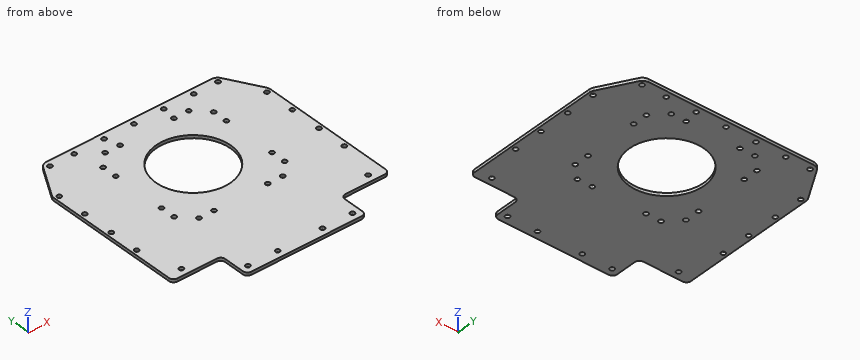
```python
from build123d import *

# Parameters (mm, degrees)
SKETCH_1_R          = 1.5
EXTRUDE_1_DEPTH     = 2
SKETCH_2_R          = 25
CUT_EXTRUDE_1_DEPTH = 2


with BuildPart() as part:
    # 草图1 → 凸台-拉伸1 (new body)
    with BuildSketch(Plane.XY):
        with BuildLine():
            Line((-60.191772409, 67.5), (-72.512280484, 46.160254038))
            ThreePointArc((-72.512280484, 46.160254038), (-73.011782597, 44.954349263), (-73.182153465, 43.660254038))
            Line((-73.182153465, 43.660254038), (-73.182153465, -47))
            ThreePointArc((-73.182153465, -47), (-72.303473809, -49.121320344), (-70.182153465, -50))
            Line((-70.182153465, -50), (-43.682153465, -50))
            ThreePointArc((-43.682153465, -50), (-41.560833122, -50.878679656), (-40.682153465, -53))
            Line((-40.682153465, -53), (-40.682153465, -67))
            ThreePointArc((-40.682153465, -67), (-39.803473809, -69.121320344), (-37.682153465, -70))
            Line((-37.682153465, -70), (36.317846535, -70))
            ThreePointArc((36.317846535, -70), (38.439166878, -69.121320344), (39.317846535, -67))
            Line((39.317846535, -67), (39.317846535, -53))
            ThreePointArc((39.317846535, -53), (40.196526191, -50.878679656), (42.317846535, -50))
            Line((42.317846535, -50), (68.817846535, -50))
            ThreePointArc((68.817846535, -50), (70.939166878, -49.121320344), (71.817846535, -47))
            Line((71.817846535, -47), (71.817846535, 43.660254038))
            ThreePointArc((71.817846535, 43.660254038), (71.647475666, 44.954349263), (71.147973554, 46.160254038))
            Line((71.147973554, 46.160254038), (58.827465478, 67.5))
            ThreePointArc((58.827465478, 67.5), (56.997338459, 69.330127019), (54.497338459, 70))
            Line((54.497338459, 70), (-55.86164539, 70))
            ThreePointArc((-55.86164539, 70), (-58.36164539, 69.330127019), (-60.191772409, 67.5))
        make_face()
        with Locations((-0.682153465, 66)):
            Circle(SKETCH_1_R, mode=Mode.SUBTRACT)
        with Locations((-20.682153465, 66)):
            Circle(SKETCH_1_R, mode=Mode.SUBTRACT)
        with Locations((19.317846535, 66)):
            Circle(SKETCH_1_R, mode=Mode.SUBTRACT)
        with Locations((39.317846535, 66)):
            Circle(SKETCH_1_R, mode=Mode.SUBTRACT)
        with Locations((55.567846535, 66)):
            Circle(SKETCH_1_R, mode=Mode.SUBTRACT)
        with Locations((68.817846535, 43)):
            Circle(SKETCH_1_R, mode=Mode.SUBTRACT)
        with Locations((68.817846535, 23)):
            Circle(SKETCH_1_R, mode=Mode.SUBTRACT)
        with Locations((68.817846535, 2)):
            Circle(SKETCH_1_R, mode=Mode.SUBTRACT)
        with Locations((68.817846535, -18)):
            Circle(SKETCH_1_R, mode=Mode.SUBTRACT)
        with Locations((61.817846535, -45)):
            Circle(SKETCH_1_R, mode=Mode.SUBTRACT)
        with Locations((34.317846535, -65)):
            Circle(SKETCH_1_R, mode=Mode.SUBTRACT)
        with Locations((14.317846535, -65)):
            Circle(SKETCH_1_R, mode=Mode.SUBTRACT)
        with Locations((-15.682153465, -65)):
            Circle(SKETCH_1_R, mode=Mode.SUBTRACT)
        with Locations((-35.682153465, -65)):
            Circle(SKETCH_1_R, mode=Mode.SUBTRACT)
        with Locations((-63.182153465, -45)):
            Circle(SKETCH_1_R, mode=Mode.SUBTRACT)
        with Locations((-70.182153465, -18)):
            Circle(SKETCH_1_R, mode=Mode.SUBTRACT)
        with Locations((-70.182153465, 2)):
            Circle(SKETCH_1_R, mode=Mode.SUBTRACT)
        with Locations((-70.182153465, 23)):
            Circle(SKETCH_1_R, mode=Mode.SUBTRACT)
        with Locations((-70.182153465, 43)):
            Circle(SKETCH_1_R, mode=Mode.SUBTRACT)
        with Locations((-40.682153465, 66)):
            Circle(SKETCH_1_R, mode=Mode.SUBTRACT)
        with Locations((-56.932153465, 66)):
            Circle(SKETCH_1_R, mode=Mode.SUBTRACT)
        with Locations((-37.005212206, 37.538233198)):
            Circle(SKETCH_1_R, mode=Mode.SUBTRACT)
        with Locations((17.994787794, 56.538233198)):
            Circle(SKETCH_1_R, mode=Mode.SUBTRACT)
        with Locations((27.994787794, 56.538233198)):
            Circle(SKETCH_1_R, mode=Mode.SUBTRACT)
        with Locations((36.994787794, 47.538233198)):
            Circle(SKETCH_1_R, mode=Mode.SUBTRACT)
        with Locations((36.994787794, 37.538233198)):
            Circle(SKETCH_1_R, mode=Mode.SUBTRACT)
        with Locations((36.994787794, 1.538233198)):
            Circle(SKETCH_1_R, mode=Mode.SUBTRACT)
        with Locations((36.994787794, -8.461766802)):
            Circle(SKETCH_1_R, mode=Mode.SUBTRACT)
        with Locations((27.994787794, -17.461766802)):
            Circle(SKETCH_1_R, mode=Mode.SUBTRACT)
        with Locations((17.994787794, -17.461766802)):
            Circle(SKETCH_1_R, mode=Mode.SUBTRACT)
        with Locations((-18.005212206, -17.461766802)):
            Circle(SKETCH_1_R, mode=Mode.SUBTRACT)
        with Locations((-28.005212206, -17.461766802)):
            Circle(SKETCH_1_R, mode=Mode.SUBTRACT)
        with Locations((-37.005212206, -8.461766802)):
            Circle(SKETCH_1_R, mode=Mode.SUBTRACT)
        with Locations((-37.005212206, 1.538233198)):
            Circle(SKETCH_1_R, mode=Mode.SUBTRACT)
        with Locations((-18.005212206, 56.538233198)):
            Circle(SKETCH_1_R, mode=Mode.SUBTRACT)
        with Locations((-28.005212206, 56.538233198)):
            Circle(SKETCH_1_R, mode=Mode.SUBTRACT)
        with Locations((-37.005212206, 47.538233198)):
            Circle(SKETCH_1_R, mode=Mode.SUBTRACT)
    extrude(amount=EXTRUDE_1_DEPTH)

    # 草图2 → 切除-拉伸1 (cut)
    with BuildSketch(Plane.XY.offset(2)):
        with Locations((0, 20)):
            Circle(SKETCH_2_R)
    extrude(amount=-CUT_EXTRUDE_1_DEPTH, mode=Mode.SUBTRACT)


solid = part.part
```
For this review, take the finished solid that the model builds, in its own axes (mm). Round coordinates to 2 decimals unless told otherwise and drop trailing zeros. Write each loop counter-clockwise with the first axis right and the second up, starting at its lowest first coordinate (ties: lowest second). Pieces come first, ordered by that corner, then holes. Notation, with made-up numbers: (-38.75, 26.5) - (8.25, 26.5) arc R21 ccw to (8.25, 54.5) - close; hole circle Ø7 at (46.5, 81). An arc over 180 degrees is marked (long way). Answer as a JSON object with one key per item and string values.
1. For pin 1 Ø1.8 at (x, y) = (68.82, 2) entering from +Z, flat-tipped, find the tip position at first contact; note if it passes through.
Response values:
{"pin 1": "passes through"}
2. To check wall thickness, follow line 1 along X through (y, z) = (-65, 1.3); line 2 along Y through (x, z) = (-14.5, 1.25); line 3 along Y through (x, z) = (54, 0.6). State the ranges of each line that lie inside material, in increasing order.
Response values:
{"line 1": "x = -40.68 to -37.18, -34.18 to -17.18, -14.18 to 12.82, 15.82 to 32.82, 35.82 to 39.32", "line 2": "y = -70 to -65.92, -64.08 to -0.37, 40.37 to 70", "line 3": "y = -50 to 70"}
3. We need section B-B on z = 1.1. Count the separate pieces of the cut face and the enclosed holes in it, then the cut area to 3 significant figures.
Response values:
{"separate pieces": "1", "enclosed holes": "38", "area": "16,400 mm2"}
4. We need section C-C on x = 51. Give the boundary of the cut face in (y, z).
Response values:
{"outline": "(-50, 0) - (70, 0) - (70, 2) - (-50, 2) - close"}
5. We need section A-A on x = -6.5. Give the boundary of the cut face in (y, z), then the cut area to 3 significant figures.
Response values:
{"outline": "(-70, 0) - (-4.14, 0) - (-4.14, 2) - (-70, 2) - close; (44.14, 0) - (70, 0) - (70, 2) - (44.14, 2) - close", "area": "183 mm2"}
